For this review, use the dimensioned drawing (mm, ordinates from the lowest corner) and the shaded views. Round coordinates to 2 decimals unless told otherwise and drop trailing zeros. Loops run counter-clockwise (first coordinate to the right, second up) from the corner with the lowest first, then second, coordinate; pieces in that order, holes last. Notation, with made-up numbers: M 63.25,67.25 L 70.25,67.25 A25 cw 70.25,102.25 Z; hole C 41.5,43.5 d10. An arc over 180 degrees is marked long. Write item = value, one per line. Start each with the question number.
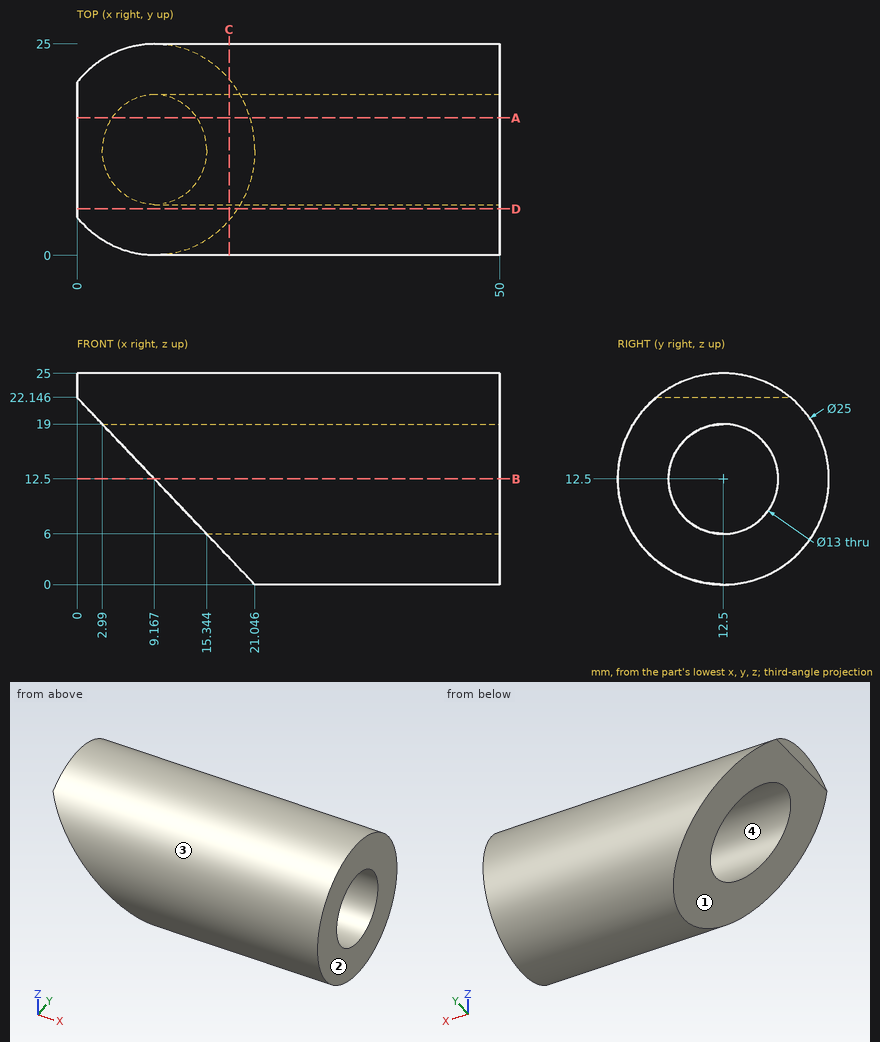
(1) Add section D-D on y = 5.5. Write out the cut boundary in (x, z).
(2) Draft analysis for pull direction Z (two halves, no side actions). For the marked faces 1, 2, 3 and 4, state which applies: +Z half, -Z half, draft (parallel to the pull), parting line (faces both ways), or undercut.
(3) Add section A-A on y = 16.25. Write out the cut boundary in (x, z), and give its area (3 significant figures).
(4) Add section B-B on z = 12.5. Write out the cut boundary in (x, y).
(5) Add section C-C on x = 18. Write out the cut boundary in (y, z) (1 decimal), and give its area (3 significant figures).
(6) For pin 1 Ø1 at (x, y) = (25, 14.5) entering from +Z; pin 2 Ø8 at (x, z) = (13.5, 6.5) entering from -Y; pin 3 Ø1.5 at (x, y) = (33, 15) entering from -Z, all flat-tipped, find the tip position at first contact; note any pin that passes through.
(7) Wall thickness on L1, parallel to Z at x = 35, y = 12.5; L2, parallel to Z at x = 17.5, y = 12.5: over which ranges is each line inside the solid? List them lowest first.
Answer sheet:
q1.outline = M 0,22.15 L 19.01,2.14 L 50,2.14 L 50,22.86 L 0,22.86 Z
q2.face_1 = -Z half
q2.face_2 = draft
q2.face_3 = parting line
q2.face_4 = undercut
q3.outline = M 0,22.15 L 4.12,17.81 L 50,17.81 L 50,24.42 L 0,24.42 Z; M 14.21,7.19 L 20.5,0.58 L 50,0.58 L 50,7.19 Z
q3.area = 538 mm²
q4.outline = M 9.17,0 L 50,0 L 50,6 L 9.17,6 Z; M 9.17,19 L 50,19 L 50,25 L 9.17,25 Z
q5.outline = M 4.1,3.2 L 20.9,3.2 A12.5 ccw long Z; hole C 12.5,12.5 d13
q5.area = 321 mm²
q6.pin_1 = 24.91
q6.pin_2 = 0.16
q6.pin_3 = 0.12
q7.L1 = 0 to 6, 19 to 25
q7.L2 = 3.73 to 6, 19 to 25
